```python
from build123d import *

# Parameters (mm, degrees)
SKETCH1_W           = 41.514809608
SKETCH1_H           = 98.81
SKETCH1_R           = 1.8288
SKETCH1_R_2         = 2.413
BOSS_EXTRUDE1_DEPTH = 3.175
CUT_EXTRUDE1_DEPTH  = 106.912542124
FILLET1_R           = 2.5
FILLET2_R           = 5


with BuildPart() as part:
    # Sketch1 → Boss-Extrude1 (new body)
    # profile 1 of 2: a face of its own
    with BuildSketch(Plane(origin=(0, 0, 0), x_dir=(0, 0, -1), z_dir=(1, 0, 0))):
        with Locations((0, -54.405)):
            Rectangle(SKETCH1_W, SKETCH1_H)
        with Locations((13.4747, -100)):
            Circle(SKETCH1_R, mode=Mode.SUBTRACT)
        with Locations((-13.4747, -100)):
            Circle(SKETCH1_R, mode=Mode.SUBTRACT)
    # profile 2 of 2: a face of its own
    with BuildSketch(Plane(origin=(0, 0, 0), x_dir=(0, 0, -1), z_dir=(1, 0, 0))):
        Polygon((0, 48.916537522), (20.757404804, -5), (-20.757404804, -5), align=None)
        with Locations((13.4747, 0)):
            Circle(SKETCH1_R, mode=Mode.SUBTRACT)
        with Locations((0, 35)):
            Circle(SKETCH1_R_2, mode=Mode.SUBTRACT)
        with Locations((-13.4747, 0)):
            Circle(SKETCH1_R, mode=Mode.SUBTRACT)
    extrude(amount=BOSS_EXTRUDE1_DEPTH)

    # Sketch2 → Cut-Extrude1 (cut, through all)
    with BuildSketch(Plane(origin=(3.175, 0, 0), x_dir=(0, 0, -1), z_dir=(1, 0, 0))):
        Polygon((16.645, 5.681808734), (16.645, -103.81), (20.757404804, -103.81), (20.757404804, -5), align=None)
        Polygon((-20.757404804, -103.81), (-16.645, -103.81), (-16.645, 5.681808734), (-20.757404804, -5), align=None)
        Polygon((-11.645, -91.821329309), (-2.784341903, -73.75), (-11.645, -55.678670691), align=None)
        Polygon((8.860658097, -97.5), (0, -79.428670691), (-8.860658097, -97.5), align=None)
        Polygon((2.784341903, -73.75), (11.645, -91.821329309), (11.645, -55.678670691), align=None)
        Polygon((-8.860658097, -50), (0, -68.071329309), (8.860658097, -50), (0, -31.928670691), align=None)
        Polygon((11.645, -8.178670691), (2.784341903, -26.25), (11.645, -44.321329309), align=None)
        Polygon((-11.645, -44.321329309), (-2.784341903, -26.25), (-11.645, -8.178670691), align=None)
        Polygon((-8.860658097, -2.5), (0, -20.571329309), (8.860658097, -2.5), align=None)
    extrude(amount=-CUT_EXTRUDE1_DEPTH, mode=Mode.SUBTRACT)

    # Fillet1
    fillet1_edges = [part.edges().sort_by_distance(p)[0] for p in [
        (1.5875, -91.821329309, -11.645),
        (1.5875, -73.75, -2.784341903),
        (1.5875, -55.678670691, -11.645),
        (1.5875, -97.5, 8.860658097),
        (1.5875, -79.428670691, 0),
        (1.5875, -97.5, -8.860658097),
        (1.5875, -103.81, -16.645),
        (1.5875, -44.321329309, -11.645),
        (1.5875, -26.25, -2.784341903),
        (1.5875, -8.178670691, -11.645),
        (1.5875, -50, -8.860658097),
        (1.5875, -68.071329309, 0),
        (1.5875, -50, 8.860658097),
        (1.5875, -31.928670691, 0),
        (1.5875, -2.5, -8.860658097),
        (1.5875, -20.571329309, 0),
        (1.5875, -2.5, 8.860658097),
        (1.5875, -8.178670691, 11.645),
        (1.5875, -26.25, 2.784341903),
        (1.5875, -44.321329309, 11.645),
        (1.5875, -103.81, 16.645),
        (1.5875, -55.678670691, 11.645),
        (1.5875, -73.75, 2.784341903),
        (1.5875, -91.821329309, 11.645),
    ]]
    fillet(fillet1_edges, radius=FILLET1_R)

    # Fillet2
    fillet2_edges = [part.edges().sort_by_distance(p)[0] for p in [
        (1.5875, 48.916537522, 0),
        (1.5875, 5.681808734, -16.645),
        (1.5875, 5.681808734, 16.645),
    ]]
    fillet(fillet2_edges, radius=FILLET2_R)


solid = part.part
```
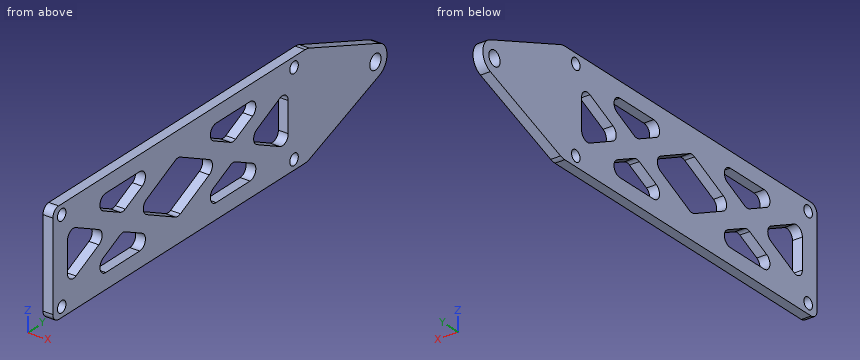
Work out the finished part from the listing and answer in its coordinate system (mm). Coordinates: 2 decimals unless noted, no trailing zeros. Write each loop counter-clockwise with the first axis right and the second up, starting at its lowest first coordinate (ties: lowest second). Pieces come first, ordered by that corner, then holes.
Q1. Each of these flat-tipped pins is pushed along its axis until it touches: pin 1 Ø3 at (y, z) = (0, -13.47) entering from -X; pin 2 Ø1.6 at (x, z) = (1, -2.5) entering from +Y. Where does it stop, or does it pass through?
Q2. A cutting plane is placed at B-B, the plane z = 0. Give the vertices of the cut face in (x, y) (3 decimals).
Q3. A cutting plane is placed at C-C, the plane z = 10. Give the vertices of the cut face in (x, y) (3 decimals), then the cut area to 3 significant figures.
Q4. A cutting plane is placed at D-D, the plane y = 35. Give the vertices of the cut face in (x, z) (3 decimals), then the cut area to 3 significant figures.
Q5. A cutting plane is placed at A-A, the plane y = -100. Give the vertices of the cut face in (x, z) (1 decimal), then the cut area to 3 significant figures.
Q6. Find the intervals of material crossed by line 1 (Z direction, x = 1.95, y = -100) (1 decimal); line 2 (Z direction, x = 1.85, y = -76.5) (3 decimals); line 3 (Y direction, x = 2.55, z = -3), in increasing order.
Findings below:
1. pin 1: passes through
1. pin 2: stops at y = 39.7
2. outline: (0, -103.81) - (3.175, -103.81) - (3.175, -97.5) - (0, -97.5) - close; (0, -82.607) - (3.175, -82.607) - (3.175, -64.893) - (0, -64.893) - close; (0, -35.107) - (3.175, -35.107) - (3.175, -17.393) - (0, -17.393) - close; (0, -2.5) - (3.175, -2.5) - (3.175, 32.587) - (0, 32.587) - close; (0, 37.413) - (3.175, 37.413) - (3.175, 40) - (0, 40) - close
3. outline: (0, -103.81) - (3.175, -103.81) - (3.175, -83.393) - (0, -83.393) - close; (0, -64.107) - (3.175, -64.107) - (3.175, -35.893) - (0, -35.893) - close; (0, -16.607) - (3.175, -16.607) - (3.175, 22.942) - (0, 22.942) - close
3. area: 280 mm2
4. outline: (0, -5.358) - (3.175, -5.358) - (3.175, -2.413) - (0, -2.413) - close; (0, 2.413) - (3.175, 2.413) - (3.175, 5.358) - (0, 5.358) - close
4. area: 18.7 mm2
5. outline: (0, -16.6) - (3.2, -16.6) - (3.2, -15.3) - (0, -15.3) - close; (0, -11.6) - (3.2, -11.6) - (3.2, 11.6) - (0, 11.6) - close; (0, 15.3) - (3.2, 15.3) - (3.2, 16.6) - (0, 16.6) - close
5. area: 82.5 mm2
6. line 1: z = -16.6 to -15.3, -11.6 to 11.6, 15.3 to 16.6
6. line 2: z = -16.645 to -11.645, -4.133 to 4.133, 11.645 to 16.645
6. line 3: y = -103.81 to -97.5, -85.55 to -61.95, -38.05 to -14.45, -2.5 to 39
